Geometry: final body of the model. Coordinates: model frame, mm. Face numbers are marked on the shaded views. A direction names the side the tool comes from. Coordinates: 2 decimals unless noted, no trailing zeros. Order: outer loops, then holes, each group sorted by start corner. A loop starts at its lowest first (then second) coordinate and runs counter-clockwise, first axis right, second up. Notation, with made-up numbers: M 73.25,58.5 L 81.25,58.5 A13 ccw 81.25,64.5 Z; hole C 54.5,36 d5. An arc over 180 degrees is marked long. Write item = value, one per line. Start each with the question number.
```python
from build123d import *

# Parameters (mm, degrees)
BOSS_EXTRU_1_DEPTH           = 7.5
BOSS_EXTRU_1_DEPTH_BACK      = 7.5
ENL_V_MAT_EXTRU_1_DEPTH      = 7.5
CONG_1_R                     = 10
CONG_2_R                     = 10
ENL_V_MAT_EXTRU_3_DEPTH      = 100.278648258
ENL_V_MAT_EXTRU_3_DEPTH_BACK = 100.278648258
ENL_V_MAT_EXTRU_2_DEPTH      = 100.278648258
ENL_V_MAT_EXTRU_2_DEPTH_BACK = 100.278648258
ESQUISSE8_R                  = 1.5
ENL_V_MAT_EXTRU_4_DEPTH      = 100.278648258


with BuildPart() as part:
    # Esquisse1 → Boss.-Extru.1 (new, two sides: drawn at the far end of the back side and taken through both)
    with BuildSketch(Plane.XY.offset(-BOSS_EXTRU_1_DEPTH_BACK)):
        Polygon((-62.45, 0), (-70, 0), (-70, -30), (-40, -70), (0, -70), (0, 0), (-27.55, 0), (-27.55, 22.5), (-62.45, 22.5), align=None)
    extrude(amount=BOSS_EXTRU_1_DEPTH + BOSS_EXTRU_1_DEPTH_BACK)

    # Esquisse3 → Enlèv. mat.-Extru.1 (cut)
    with BuildSketch(Plane.XY):
        Polygon((-32.65, 0), (-32.65, 7.5), (-57.35, 7.5), (-57.35, 0), (-62.45, 0), (-62.45, 22.5), (-27.55, 22.5), (-27.55, 0), align=None)
    extrude(amount=ENL_V_MAT_EXTRU_1_DEPTH, mode=Mode.SUBTRACT)

    # Congé1
    # the kernel refuses this fillet: 10 mm, written as the material it takes off along each edge
    with BuildSketch(Plane(origin=(-62.45, 22.5, 25), x_dir=(1, 0, 0), z_dir=(0, 0, -1))) as cong_1_piece_1:
        with BuildLine():
            CenterArc((CONG_1_R, CONG_1_R), CONG_1_R, 180, 90)
            Line((0, CONG_1_R), (0, 0))
            Line((0, 0), (CONG_1_R, 0))
        make_face()
    extrude(amount=57.5, mode=Mode.SUBTRACT)
    with BuildSketch(Plane(origin=(-57.35, 7.5, 0), x_dir=(1, 0, 0), z_dir=(0, 0, 1))) as cong_1_piece_2:
        with BuildLine():
            CenterArc((9.682458366, -10), CONG_1_R, 90, 75.522487814)
            Line((0, -7.5), (0, 0))
            Line((0, 0), (9.682458366, 0))
        make_face()
    extrude(amount=31.706145914, mode=Mode.SUBTRACT)
    with BuildSketch(Plane(origin=(-32.65, 7.5, 0), x_dir=(0, -1, 0), z_dir=(0, 0, 1))) as cong_1_piece_3:
        with BuildLine():
            CenterArc((10, -9.682458366), CONG_1_R, 104.477512186, 75.522487814)
            Line((0, -9.682458366), (0, 0))
            Line((0, 0), (7.5, 0))
        make_face()
    extrude(amount=31.706145914, mode=Mode.SUBTRACT)
    with BuildSketch(Plane(origin=(-27.55, 22.5, 25), x_dir=(-1, 0, 0), z_dir=(0, 0, -1))) as cong_1_piece_4:
        with BuildLine():
            CenterArc((CONG_1_R, -CONG_1_R), CONG_1_R, 90, 90)
            Line((0, -CONG_1_R), (0, 0))
            Line((0, 0), (CONG_1_R, 0))
        make_face()
    extrude(amount=57.5, mode=Mode.SUBTRACT)

    # Congé2
    cong_2_edges = [part.edges().sort_by_distance(p)[0] for p in [
        (-40, -70, 0),
        (-70, -30, 0),
    ]]
    fillet(cong_2_edges, radius=CONG_2_R)

    # Esquisse6 → Enlèv. mat.-Extru.3 (cut, two sides: drawn at the far end of the back side and taken through both)
    with BuildSketch(Plane.XY.offset(-ENL_V_MAT_EXTRU_3_DEPTH_BACK)):
        with BuildLine():
            Line((-58, -22), (-58, -22.666666667))
            ThreePointArc((-58, -22.666666667), (-57.486832981, -25.828944327), (-56, -28.666666667))
            Line((-56, -28.666666667), (-43, -46))
            ThreePointArc((-43, -46), (-39.472135955, -48.94427191), (-35, -50))
            Line((-35, -50), (-22, -50))
            ThreePointArc((-22, -50), (-14.928932188, -47.071067812), (-12, -40))
            Line((-12, -40), (-12, -22))
            ThreePointArc((-12, -22), (-14.928932188, -14.928932188), (-22, -12))
            Line((-22, -12), (-48, -12))
            ThreePointArc((-48, -12), (-55.071067812, -14.928932188), (-58, -22))
        make_face()
    extrude(amount=ENL_V_MAT_EXTRU_3_DEPTH + ENL_V_MAT_EXTRU_3_DEPTH_BACK, mode=Mode.SUBTRACT)

    # Esquisse5 → Enlèv. mat.-Extru.2 (cut, two sides: drawn at the far end of the back side and taken through both)
    with BuildSketch(Plane.XY.offset(-ENL_V_MAT_EXTRU_2_DEPTH_BACK)):
        with BuildLine():
            Line((-29, -72.5), (-31, -72.5))
            Line((-31, -72.5), (-31, -63.769615365))
            ThreePointArc((-31, -63.769615365), (-33.9, -60), (-31, -56.230384635))
            Line((-31, -56.230384635), (-31, -47.5))
            Line((-31, -47.5), (-29, -47.5))
            Line((-29, -47.5), (-29, -56.230384635))
            ThreePointArc((-29, -56.230384635), (-26.1, -60), (-29, -63.769615365))
            Line((-29, -63.769615365), (-29, -72.5))
        make_face()
    extrude(amount=ENL_V_MAT_EXTRU_2_DEPTH + ENL_V_MAT_EXTRU_2_DEPTH_BACK, mode=Mode.SUBTRACT)

    # Esquisse8 → Enlèv. mat.-Extru.4 (cut, through all)
    with BuildSketch(Plane.XY):
        with Locations((-55, 14.5)):
            Circle(ESQUISSE8_R)
        with Locations(Location((-35, 14.5, 0), (0, 0, 180))):
            Circle(ESQUISSE8_R)
    extrude(amount=-ENL_V_MAT_EXTRU_4_DEPTH, mode=Mode.SUBTRACT)

    # Symétrie1: part across plane


with BuildPart() as part_1:
    add(part.part)
    add(part.part.mirror(Plane(origin=(0, 0, -7.5), x_dir=(0, 0, 1), z_dir=(1, 0, 0))))


solid = part_1.part
```
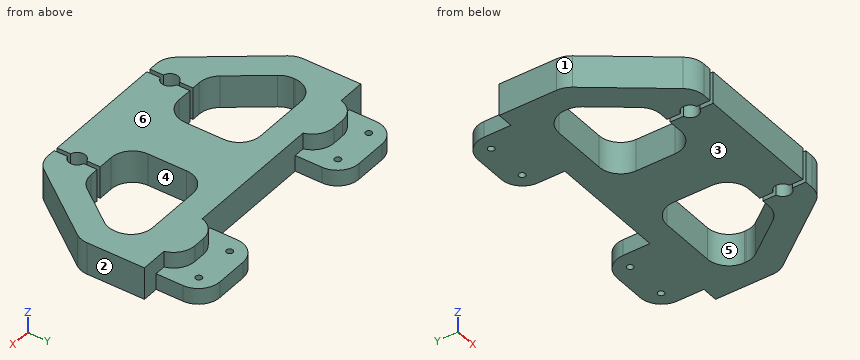
Item 1: Section query A-A on y = -35. Output: boundary loops of the cut face in (x, z), and give its area (3 significant figures).
Item 2: Draft query along X for the marked faces 1, 2, 3 and 4. Return one class per face: pulls with the +X half, pulls with the -X half, needs draft (parallel to the pull), parting line crosses it, or undercut.
Item 3: Section query C-C on x = -7.5. Output: boundary loops of the cut face in (y, z), and give its area (3 significant figures).
Item 4: Material intervals for probe 1 along X at (y, z) = (-40, 4); probe 2 along Y at (x, z) = (41, -3); probe 3 along X at (y, z) = (-45.5, -2.5) (3 decimals), sorted ascending. Write a range as [from, to].
Item 5: Reachability of the marked faces 5 and 6 from +Z, -Z, +X, -X, +Y, -Y: full face, straight path, thin tool, end or side. Return the list, or none.
Item 6: First-contact query: pin 1 (7 mm diameter, centred on y = -54.5, z = -2.5, fed in from -X); pin 2 (4 mm diameter, centred on y = 7.5, z = -3.5, fed in from +X); pin 3 (2.5 mm diameter, centred on x = 44.5, z = 3, fed in from +Y). Flat tips, straight axial feed; report the tip coordinate or a pass-through.
Item 7: Section query B-B on y = 9. Output: boundary loops of the cut face in (x, z).
Ans:
q1.outline = M -66.25,-7.5 L -51.25,-7.5 L -51.25,7.5 L -66.25,7.5 Z; M -12,-7.5 L 12,-7.5 L 12,7.5 L -12,7.5 Z; M 51.25,-7.5 L 66.25,-7.5 L 66.25,7.5 L 51.25,7.5 Z
q1.area = 810 mm^2
q2.face_1 = pulls with the -X half
q2.face_2 = pulls with the +X half
q2.face_3 = needs draft
q2.face_4 = undercut
q3.outline = M -70,-7.5 L 0,-7.5 L 0,7.5 L -70,7.5 Z
q3.area = 1,050 mm^2
q4.probe_1 = [-62.5, -47.5], [-12, 12], [47.5, 62.5]
q4.probe_2 = [-68, -48], [-12, 22.5]
q4.probe_3 = [-58.375, -43.375], [-13.648, 13.648], [43.375, 58.375]
q5.face_5 = +Z, -Z
q5.face_6 = +Z, +X, -X, +Y, -Y
q6.pin_1 = -54.25
q6.pin_2 = 62.45
q6.pin_3 = 7.5
q7.outline = M -62.45,-7.5 L -27.55,-7.5 L -27.55,0 L -62.45,0 Z; M 27.55,-7.5 L 62.45,-7.5 L 62.45,0 L 27.55,0 Z
